Geometry: final body of the model. Coordinates: model frame, mm. Face numbers are marked on the shaded views. A direction names the side the tool comes from. Coordinates: 2 decimals unless noted, no trailing zeros. Write each loop counter-clockwise with the first axis right and the second up, starting at its lowest first coordinate (ties: lowest second). Pieces come first, ordered by that corner, then holes.
from build123d import *

# Parameters (mm, degrees)
F0_R     = 2.875
F1_DEPTH = 8
F2_DEPTH = 4
F3_DEPTH = 19
F4_R     = 3.25
F5_DEPTH = 25


with BuildPart() as f1:
    # F0 (on Top) → F1 (new body)
    with BuildSketch(Plane.XY):
        Circle(F0_R)
    extrude(amount=F1_DEPTH)

    # F0 (on Top) → F2 (join)
    with BuildSketch(Plane.XY):
        with BuildLine():
            ThreePointArc((-6.928203, -4), (0, -8), (6.928203, -4))
            Line((6.928203, -4), (-6.928203, -4))
        make_face()
        with BuildLine():
            Line((-6.928203, 4), (6.928203, 4))
            ThreePointArc((6.928203, 4), (0, 8), (-6.928203, 4))
        make_face()
        with BuildLine():
            ThreePointArc((6.928203, -4), (7.727407, -2.070552), (8, 0))
            ThreePointArc((8, 0), (7.727407, 2.070552), (6.928203, 4))
            Line((6.928203, 4), (-6.928203, 4))
            ThreePointArc((-6.928203, 4), (-8, 0), (-6.928203, -4))
            Line((-6.928203, -4), (6.928203, -4))
        make_face()
        Circle(F0_R, mode=Mode.SUBTRACT)
        Circle(F0_R)
    extrude(amount=-F2_DEPTH)

    # F0 (on Top) → F3 (join)
    with BuildSketch(Plane.XY):
        with BuildLine():
            ThreePointArc((6.928203, -4), (7.727407, -2.070552), (8, 0))
            ThreePointArc((8, 0), (7.727407, 2.070552), (6.928203, 4))
            Line((6.928203, 4), (-6.928203, 4))
            ThreePointArc((-6.928203, 4), (-8, 0), (-6.928203, -4))
            Line((-6.928203, -4), (6.928203, -4))
        make_face()
        Circle(F0_R, mode=Mode.SUBTRACT)
        Circle(F0_R)
    extrude(amount=-F3_DEPTH)

    # F4 (on face) → F5 (cut)
    with BuildSketch(Plane(origin=(0, 4, 0), x_dir=(-1, 0, 0), z_dir=(0, 1, 0))):
        with Locations((0, -11.5)):
            Circle(F4_R)
    extrude(amount=-F5_DEPTH, mode=Mode.SUBTRACT)


solid = f1.part
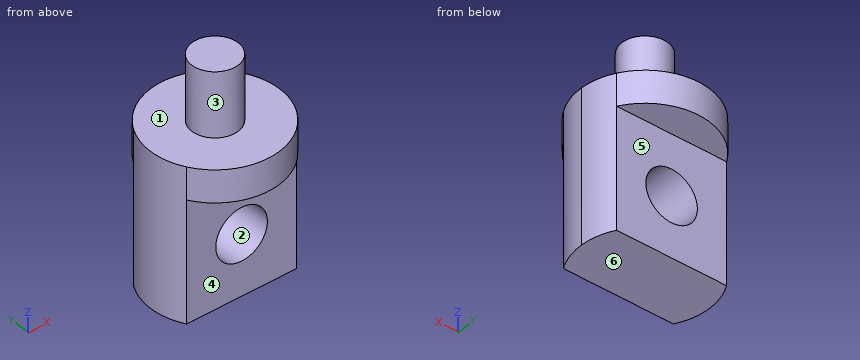
Item 1: Pull-direction query (X, two-part tool) for the marked faces 1, 2 and 3; classes: released by +X, released by -X, zero draft, split by the parting line, or undercut.
Derived:
face 1: zero draft
face 2: undercut
face 3: split by the parting line
Item 2: Section C-C, the plane y = -1.5. Output: boundary loops of the cut face in (x, z), plus the area to 3 significant figures.
Derived:
outline: (-7.86, -19) - (7.86, -19) - (7.86, 0) - (2.45, 0) - (2.45, 8) - (-2.45, 8) - (-2.45, 0) - (-7.86, 0) - close; hole circle Ø6.5 at (0, -11.5)
area: 305 mm2
Item 3: Pin query (flat end, axial travel): pin 1 (1.5 mm diameter, centred on x = -2.5, y = 5.5, fed in from -Z); pin 2 (5 mm diameter, centred on x = -3.5, z = -4, fed in from +Y); pin 3 (2 mm diameter, centred on x = -5.5, y = 0.5, fed in from +Z). Return the tip coordinate at first contact, or that it passes through.
Derived:
pin 1: stops at z = -4
pin 2: stops at y = 7.94
pin 3: stops at z = 0
Item 4: Section B-B, the plane z = -11.5. Output: boundary loops of the cut face in (x, y), plus the area to 3 significant figures.
Derived:
outline: (-6.93, -4) - (-3.25, -4) - (-3.25, 4) - (-6.93, 4) arc R8 ccw to start; (3.25, -4) - (6.93, -4) arc R8 ccw to (8, 0) arc R8 ccw to (6.93, 4) - (3.25, 4) - close
area: 70.4 mm2
Item 5: Section A-A, the plane x = 0. Output: boundary loops of the cut face in (y, z) (3 decimals), plus the area to 3 significant figures.
Derived:
outline: (-8, -4) - (-4, -4) - (-4, -8.25) - (4, -8.25) - (4, -4) - (8, -4) - (8, 0) - (2.875, 0) - (2.875, 8) - (-2.875, 8) - (-2.875, 0) - (-8, 0) - close; (-4, -19) - (4, -19) - (4, -14.75) - (-4, -14.75) - close
area: 178 mm2
Item 6: Set-up query: the marked faces 4, 5 and 6. Return all of +Z, -Z, +X, -X, +Y, -Y with unobstructed straight access to the full face (end or side cutting, diameter ignored); none if empty.
Derived:
face 4: -Z, +X, -X, -Y
face 5: -Z, +X, -X, +Y
face 6: -Z, +X, -X, +Y, -Y
Item 7: Material intervals for probe 1 along Z at (x, y) = (0, -1.5); probe 2 along Z at (x, y) = (-2.5, 6); probe 3 along Y at (x, z) = (5, -7.75), sorted ascending.
Derived:
probe 1: z = -19 to -14.75, -8.25 to 8
probe 2: z = -4 to 0
probe 3: y = -4 to 4
Item 8: Section D-D, the plane z = -7.25. Output: boundary loops of the cut face in (x, y).
Derived:
outline: (-6.93, -4) - (6.93, -4) arc R8 ccw to (8, 0) arc R8 ccw to (6.93, 4) - (-6.93, 4) arc R8 ccw to start
